The model under review builds one solid part; all positions refer to its coordinate system, in mm. A direction names the side the tool comes from. Round coordinates to 2 decimals unless told otherwise and drop trailing zeros. Write each loop counter-clockwise with the first axis right and the second up, starting at its lowest first coordinate (ties: lowest second). Pieces come first, ordered by that corner, then holes. Notation, with made-up numbers: M 41,-6 L 89,-6 A22 ccw 89,8 Z; hole C 27.5,78 d8. An arc over 180 degrees is marked long. One line per item, written item: value. Start each with the question number.
1) Take a section at B-B, the plane x = -20. Write out the cut boundary in (y, z), and give its area (3 significant figures).
2) Take a section at C-C, the plane y = 36. Write out the cut boundary in (x, z), and give its area (3 significant figures).
3) Take a section at D-D, the plane z = 28. Write out the cut boundary in (x, y).
4) Mouldability with a two-part tool opening along X and no side actions: class faces 3 (the face through (-53.073, -1, 13)), 4 (the face through (30.916, -1.932, 12.522)), 5 (the face through (-1, 1, 25.4)) as +X half, -X half, draft (parallel to the pull), parting line (faces both ways), or undercut.
5) Wall thickness on probe 1 along Z at (x, y) = (18.5, 32.5); probe 2 along X at (y, z) = (-23, 29); probe 3 along Y at (x, z) = (-11, 45): over which ranges is each line inside the solid? List them lowest first.
6) Take a section at A-A, the plane y = 0. Write out the cut boundary in (x, z), and give its area (3 significant figures).
7) For P1, Ø8.5, axis at x = 28.4, y = 0, coming from the -Z side; P2, Ø4, axis at y = -13, z = 32.5, coming from the -X side, all flat-tipped, find the tip position at first contact; note any pin that passes through.
8) Tool access review of faces 1 (the face through (-34.275, -22.179, 37.922)), 2 (the face through (-22, -23, 50.8)): name each direction out of +Z, -Z, +X, -X, +Y, -Y from which nothing blocks a thin tool from reaching the whole face with its end or side.
from build123d import *

# Parameters (mm, degrees)
F0_W     = 106.146804
F0_H     = 93.039534
F1_DEPTH = 25.4
F3_D     = 6.35
F4_R     = 12.11582
F5_DEPTH = 25.4


with BuildPart() as f1:
    # F0 (on Top) → F1 (new body)
    with BuildSketch(Plane.XY):
        Rectangle(F0_W, F0_H)
    extrude(amount=F1_DEPTH)

    # F3 (through all)
    with Locations(Plane.XY.offset(25.4)):
        with Locations((28.396336, 0)):
            Hole(F3_D / 2)

    # F4 (on face) → F5 (join)
    with BuildSketch(Plane.XY.offset(25.4)):
        with Locations((-22.170972, -22.711303)):
            Circle(F4_R)
    extrude(amount=F5_DEPTH)


solid = f1.part
Checked values:
1. outline: M -46.52,0 L 46.52,0 L 46.52,25.4 L -10.79,25.4 L -10.79,50.8 L -34.63,50.8 L -34.63,25.4 L -46.52,25.4 Z
1. area: 2,970 mm2
2. outline: M -53.07,0 L 53.07,0 L 53.07,25.4 L -53.07,25.4 Z
2. area: 2,700 mm2
3. outline: C -22.17,-22.71 d24.23
4. face 3: -X half
4. face 4: undercut
4. face 5: draft
5. probe 1: z = 0 to 25.4
5. probe 2: x = -34.28 to -10.06
5. probe 3: y = -27.4 to -18.02
6. outline: M -53.07,0 L 25.22,0 L 25.22,25.4 L -53.07,25.4 Z; M 31.57,0 L 53.07,0 L 53.07,25.4 L 31.57,25.4 Z
6. area: 2,530 mm2
7. P1: stops at z = 0
7. P2: stops at x = -31.52
8. face 1: +Z
8. face 2: +Z, +X, -X, +Y, -Y
